Autodesk Inventor part; units mm, degrees
ref_plane "YZ Plane" through (0, 0, 0) normal (1, 0, 0) x (0, 1, 0)
ref_plane "XZ Plane" through (0, 0, 0) normal (0, 1, 0) x (-1, 0, 0)
ref_plane "XY Plane" through (0, 0, 0) normal (0, 0, 1) x (1, 0, 0)
sketch "Sketch1" plane through (0, 0, 0) normal (1, 0, 0) x (0, 1, 0)
  circle A0 centre (0, -40) radius 30.1625 construction
  line L0 (31.75, 0) -> (-31.75, 0)
  line L1 (-31.75, 0) -> (-31.75, -25.4)
  line L2 (31.75, -25.4) -> (31.75, 0)
  line L3 (0, 0) -> (0, -115.458)
  arc A1 (26.3935, -25.4) -> (-26.3935, -25.4) centre (0, -40) ccw
  line L4 (-31.75, -25.4) -> (-26.3935, -25.4)
  line L5 (26.3935, -25.4) -> (31.75, -25.4)
  dimension "d1" = 60.325
  dimension "d3" = 63.5
  dimension "d4" = 40
  dimension "d5" = 25.4
extrude "Extrusion1" add sketch "Sketch1" along normal mid plane 76.2
sketch "Sketch2" plane through (-38.1, -31.75, 0) normal (0, 0, 1) x (1, 0, 0)
  circle A0 centre (38.1, 31.75) radius 50
  dimension "d8" = 100
extrude "Extrusion2" add sketch "Sketch2" against normal blind 9
sketch "Sketch3" plane through (0, 0, 0) normal (0, 0, 1) x (1, 0, 0)
  circle A0 centre (0, 0) radius 10
  dimension "d11" = 20
extrude "Extrusion3" cut sketch "Sketch3" against normal through all
sketch "Sketch5" plane through (0, 0, 0) normal (0, 0, 1) x (1, 0, 0)
  line L0 (0, 0) -> (0, 29.874) construction
  line L1 (-38.1, 26.3935) -> (38.1, 26.3935) construction
  point P0 (25, 0)
  point P1 (-25, 0)
  point P2 (-25, 0)
  point P3 (25, 0)
  dimension "d23" = 50
hole "Hole1" at (25, 0, 0) at (-25, 0, 0) direction (0, 0, -1) diameter 5.5 end through all
properties part number "Hub Plate" material "ABS Plastic"
The model under review builds one solid part; all positions refer to its coordinate system, in mm. A direction names the side the tool comes from. Round coordinates to 2 decimals unless told otherwise and drop trailing zeros. Order: outer loops, then holes, each group sorted by start corner. A loop starts at its lowest first (then second) coordinate and runs counter-clockwise, first axis right, second up. Notation, with made-up numbers: (34, 32) - (72, 32) arc R33 ccw to (72, 64) - close; hole circle Ø10 at (57.25, 80). An arc over 180 degrees is marked (long way). Answer in a Markdown table with one row per item.
(1) Machinability: for faces 4 (the face through (10.4, 0.7, 0)), 5 (the face through (-27.32, -1.48, -5.05)), 6 (the face through (-1, 31.75, -17)), 7 (the face through (38.1, -8, -10)), 8 (the face through (-38.1, -8, -10)), which of the approach directions +Z, -Z, +X, -X, +Y, -Y give a long, thin tool a straight path to every point of the face, cutting with its end or side? Answer none if there is none.
Result set:
| item | result |
|---|---|
| face 4 | +Z, +X, -X, +Y, -Y |
| face 5 | +Z, -Z |
| face 6 | -Z, +X, -X, +Y |
| face 7 | -Z, +X, +Y, -Y |
| face 8 | -Z, -X, +Y, -Y |
(2) Mouldability with a two-part tool opening along X and no side actions: class faces 1 (the face through (-1, -31.75, -17)), 2 (the face through (47.69, 15.02, -4.44)), 3 (the face through (9.54, 3, -5.69)) as released by +X, released by -X, zero draft, split by the parting line, or undercut.
Result set:
| item | result |
|---|---|
| face 1 | zero draft |
| face 2 | split by the parting line |
| face 3 | undercut |
(3) For line 1 (Y direction, x = 0, z = -8); line 2 (X direction, y = 14, z = -11); line 3 (Y direction, x = 36, z = -14.25), list the stretches that pass through material, from the lowest coordinate up. Write a range as from..to.
Result set:
| item | result |
|---|---|
| line 1 | y = -50..-10, 10..50 |
| line 2 | x = -38.1..38.1 |
| line 3 | y = -31.75..-15.71, 15.71..31.75 |
(4) Take a section at A-A on x = 0. Write out the cut boundary in (y, z).
Result set:
| item | result |
|---|---|
| outline | (-50, -9) - (-31.75, -9) - (-31.75, -25.4) - (-26.39, -25.4) arc R30.16 cw to (-10, -11.54) - (-10, 0) - (-50, 0) - close; (10, -11.54) arc R30.16 cw to (26.39, -25.4) - (31.75, -25.4) - (31.75, -9) - (50, -9) - (50, 0) - (10, 0) - close |
(5) Take a section at D-D on x = 32.5. Write out the cut boundary in (y, z).
Result set:
| item | result |
|---|---|
| outline | (-38, -9) - (-31.75, -9) - (-31.75, -25.4) - (-26.39, -25.4) arc R30.16 cw to (26.39, -25.4) - (31.75, -25.4) - (31.75, -9) - (38, -9) - (38, 0) - (-38, 0) - close |
(6) Take a section at C-C on z = -22. Write out the cut boundary in (x, y), plus the area to 3 significant figures.
Result set:
| item | result |
|---|---|
| outline | (-38.1, -31.75) - (38.1, -31.75) - (38.1, -24.2) - (-38.1, -24.2) - close; (-38.1, 24.2) - (38.1, 24.2) - (38.1, 31.75) - (-38.1, 31.75) - close |
| area | 1,150 mm2 |
(7) Take a section at B-B on y = 0. Write out the cut boundary in (x, z), plus the area to 3 significant figures.
Result set:
| item | result |
|---|---|
| outline | (-50, -9) - (-38.1, -9) - (-38.1, -9.84) - (-27.75, -9.84) - (-27.75, 0) - (-50, 0) - close; (-22.25, -9.84) - (-10, -9.84) - (-10, 0) - (-22.25, 0) - close; (10, -9.84) - (22.25, -9.84) - (22.25, 0) - (10, 0) - close; (27.75, -9.84) - (38.1, -9.84) - (38.1, -9) - (50, -9) - (50, 0) - (27.75, 0) - close |
| area | 659 mm2 |
(8) Clearance check with flat-ended pins moving along their axes: P1, Ø8, axis at x = -20.5, z = -17.5, coming from the -Y side; P2, Ø8, axis at y = 12.5, z = -15.5, coming from the +X side; P3, Ø8, axis at x = -36, y = 1.5, coming from the +Z side; P4, Ø8, axis at x = 31.5, z = -6.5, coming from the -Y side. State where each tip first meets the part, or that it passes through.
Result set:
| item | result |
|---|---|
| P1 | stops at y = -31.75 |
| P2 | stops at x = 38.1 |
| P3 | stops at z = 0 |
| P4 | stops at y = -41.76 |
